from build123d import *

# Parameters (mm, degrees)
SKETCH1_W           = 76.2
SKETCH1_H           = 50.8
BOSS_EXTRUDE1_DEPTH = 4.572
SKETCH2_R           = 8.73125
CUT_EXTRUDE7_DEPTH  = 92.695055396
SKETCH5_R           = 1.5875
CUT_EXTRUDE8_DEPTH  = 92.695055396
CAVITY1_START       = 10.16
CAVITY1_OUTLINE_W   = 6.35
CAVITY1_OUTLINE_H   = 4.572
CAVITY1_DEPTH       = 10.16
CAVITY1_START_2     = 30.48
CAVITY1_2_OUTLINE_W = 6.35
CAVITY1_2_OUTLINE_H = 4.572
CAVITY1_2_DEPTH     = 10.16


# Read off the part's stored shape, not the designer's step: Cavity1
with BuildPart() as part:
    # Sketch1 → Boss-Extrude1 (new body)
    with BuildSketch(Plane.XY):
        with Locations((38.1, 25.4)):
            Rectangle(SKETCH1_W, SKETCH1_H)
    extrude(amount=BOSS_EXTRUDE1_DEPTH)

    # Sketch2 → Cut-Extrude7 (cut, through all)
    with BuildSketch(Plane(origin=(0, 0, 0), x_dir=(-1, 0, 0), z_dir=(0, 0, -1))):
        with Locations((-38.1, 25.4)):
            Circle(SKETCH2_R)
    extrude(amount=-CUT_EXTRUDE7_DEPTH, mode=Mode.SUBTRACT)

    # Sketch5 → Cut-Extrude8 (cut, through all)
    with BuildSketch(Plane(origin=(0, 0, 0), x_dir=(-1, 0, 0), z_dir=(0, 0, -1))):
        with Locations((-19.05, 44.45)):
            Circle(SKETCH5_R)
        with Locations((-19.05, 6.35)):
            Circle(SKETCH5_R)
        with Locations((-57.15, 44.45)):
            Circle(SKETCH5_R)
        with Locations((-57.15, 6.35)):
            Circle(SKETCH5_R)
    extrude(amount=-CUT_EXTRUDE8_DEPTH, mode=Mode.SUBTRACT)

    # Cavity1 outline → Cavity1 (cut)
    with BuildSketch(Plane(origin=(0, 0, 0), x_dir=(1, 0, 0), z_dir=(0, 1, 0)).offset(CAVITY1_START)):
        with Locations((3.175, -2.286)):
            Rectangle(CAVITY1_OUTLINE_W, CAVITY1_OUTLINE_H)
        with Locations((73.025, -2.286)):
            Rectangle(CAVITY1_OUTLINE_W, CAVITY1_OUTLINE_H)
    extrude(amount=CAVITY1_DEPTH, mode=Mode.SUBTRACT)

    # Cavity1 2 outline → Cavity1 2 (cut)
    with BuildSketch(Plane(origin=(0, 0, 0), x_dir=(1, 0, 0), z_dir=(0, 1, 0)).offset(CAVITY1_START_2)):
        with Locations((3.175, -2.286)):
            Rectangle(CAVITY1_2_OUTLINE_W, CAVITY1_2_OUTLINE_H)
        with Locations((73.025, -2.286)):
            Rectangle(CAVITY1_2_OUTLINE_W, CAVITY1_2_OUTLINE_H)
    extrude(amount=CAVITY1_2_DEPTH, mode=Mode.SUBTRACT)


solid = part.part
CAD build for the part. Positions are in the model's coordinates, mm. A direction names the side the tool comes from. Give positions to 0.01 mm unless a question says otherwise; leave off trailing zeros. Write each loop counter-clockwise with the first axis right and the second up, starting at its lowest first coordinate (ties: lowest second). Pieces come first, ordered by that corner, then holes. Notation, with made-up numbers: (-5, -26) -> (32, -26) arc R33 cw to (32, 2) -> close; hole circle Ø8 at (23.25, 34.5). An arc over 180 degrees is marked (long way). Return JSON: item names as keys, results as strings.
Item 1: Two-plate mould, pull along X, no slides. Class faces 1 (the cylindrical face through (57.5, 42.9, 2.3)), 2 (the flat face through (76.2, 46, 2)), 3 (the flat face through (3, 20.32, 2)): +X half, -X half, draft (parallel to the pull), parting line (faces both ways), or undercut.
Answer below:
{"face 1": "undercut", "face 2": "+X half", "face 3": "draft"}
Item 2: Band-saw the part on D-D (x = 38.1). List the corners of the cut face in (y, z), then the cut area to 3 significant figures.
Answer below:
{"outline": "(0, 0) -> (16.67, 0) -> (16.67, 4.57) -> (0, 4.57) -> close; (34.13, 0) -> (50.8, 0) -> (50.8, 4.57) -> (34.13, 4.57) -> close", "area": "152 mm2"}
Item 3: Drill centre lines: probe 1 along Y at (x, z) = (57.15, 2.2); probe 2 along X at (y, z) = (45.5, 1.4); probe 3 along X at (y, z) = (14.5, 4). Where is each one in solid material? Low to high.
Answer below:
{"probe 1": "y = 0 to 4.76, 7.94 to 42.86, 46.04 to 50.8", "probe 2": "x = 0 to 17.86, 20.24 to 55.96, 58.34 to 76.2", "probe 3": "x = 6.35 to 69.85"}
Item 4: Band-saw the part on B-B (y = 44.45). List the corners of the cut face in (x, z).
Answer below:
{"outline": "(0, 0) -> (17.46, 0) -> (17.46, 4.57) -> (0, 4.57) -> close; (20.64, 0) -> (55.56, 0) -> (55.56, 4.57) -> (20.64, 4.57) -> close; (58.74, 0) -> (76.2, 0) -> (76.2, 4.57) -> (58.74, 4.57) -> close"}
Item 5: Band-saw the part on C-C (y = 25.4). List the corners of the cut face in (x, z), then the cut area to 3 significant figures.
Answer below:
{"outline": "(0, 0) -> (29.37, 0) -> (29.37, 4.57) -> (0, 4.57) -> close; (46.83, 0) -> (76.2, 0) -> (76.2, 4.57) -> (46.83, 4.57) -> close", "area": "269 mm2"}
Item 6: Drop flat-ended pins along their axis: pin 1 (2.5 mm diameter, centred on y = 17.5, z = 3.5, fed in from +X); pin 2 (2.5 mm diameter, centred on y = 37.5, z = 3, fed in from -X). Give the stop position or say it passes through.
Answer below:
{"pin 1": "stops at x = 69.85", "pin 2": "stops at x = 6.35"}
Item 7: Tool access for faces 4 (the flat face through (73, 10.16, 2)), 5 (the flat face through (3, 30.48, 2)), 6 (the flat face through (29, 26, 4.572)): list every direction of +Z, -Z, +X, -X, +Y, -Y with a clear straight run to the whole face (end or side of a thin tool).
Answer below:
{"face 4": "+Z, -Z, +X", "face 5": "+Z, -Z, -X", "face 6": "+Z, +X, -X, +Y, -Y"}
Item 8: Band-saw the part on A-A (x = 19.05). List the corners of the cut face in (y, z).
Answer below:
{"outline": "(0, 0) -> (4.76, 0) -> (4.76, 4.57) -> (0, 4.57) -> close; (7.94, 0) -> (42.86, 0) -> (42.86, 4.57) -> (7.94, 4.57) -> close; (46.04, 0) -> (50.8, 0) -> (50.8, 4.57) -> (46.04, 4.57) -> close"}
